Design review of the part shown in the three views and the two pictorial views. Dimensions are in mm from the part's minimum x, y and z. A direction names the side the tool comes from. Give positions to 0.01 mm unless a question says otherwise; leave off trailing zeros. Order: outer loops, then holes, each group sorted by start corner. A loop starts at its lowest first (then second) coordinate and runs counter-clockwise, first axis right, second up.
Item 1: Machinability: for the marked faces 1 and 2, which of the approach directions +Z, -Z, +X, -X, +Y, -Y give a long, thin tool a straight path to every point of the face, cutting with its end or side? Answer none if there is none.
Item 2: For P1, Ø8, axis at y = 17.5, z = 5.5, coming from the -X side; P2, Ø2, axis at x = 24.5, y = 38.5, coming from the +Z side; P3, Ø2, axis at x = 40, y = 11.5, coming from the +Z side, all flat-tipped, find the tip position at first contact; note any pin that passes through.
Item 3: Consider section A-A (x = 44). Give the boundary of the cut face in (y, z), plus the area to 3 significant figures.
Item 4: Consider section C-C (z = 19.25). Give the boundary of the cut face in (x, y) (1 decimal).
Item 5: For probe 1 along Z at (x, y) = (38, 24.5); probe 2 along Z at (x, y) = (8.5, 33.5) (1 decimal); probe 3 along X at (y, z) = (21.5, 24) (1 decimal), list the stretches that pass through material, from the lowest coordinate up.
Item 6: The part is to be moulded in two halves that separate along X. For the marked faces 3, 4 and 5, say which applies: released by +X, released by -X, zero draft, split by the parting line, or undercut.
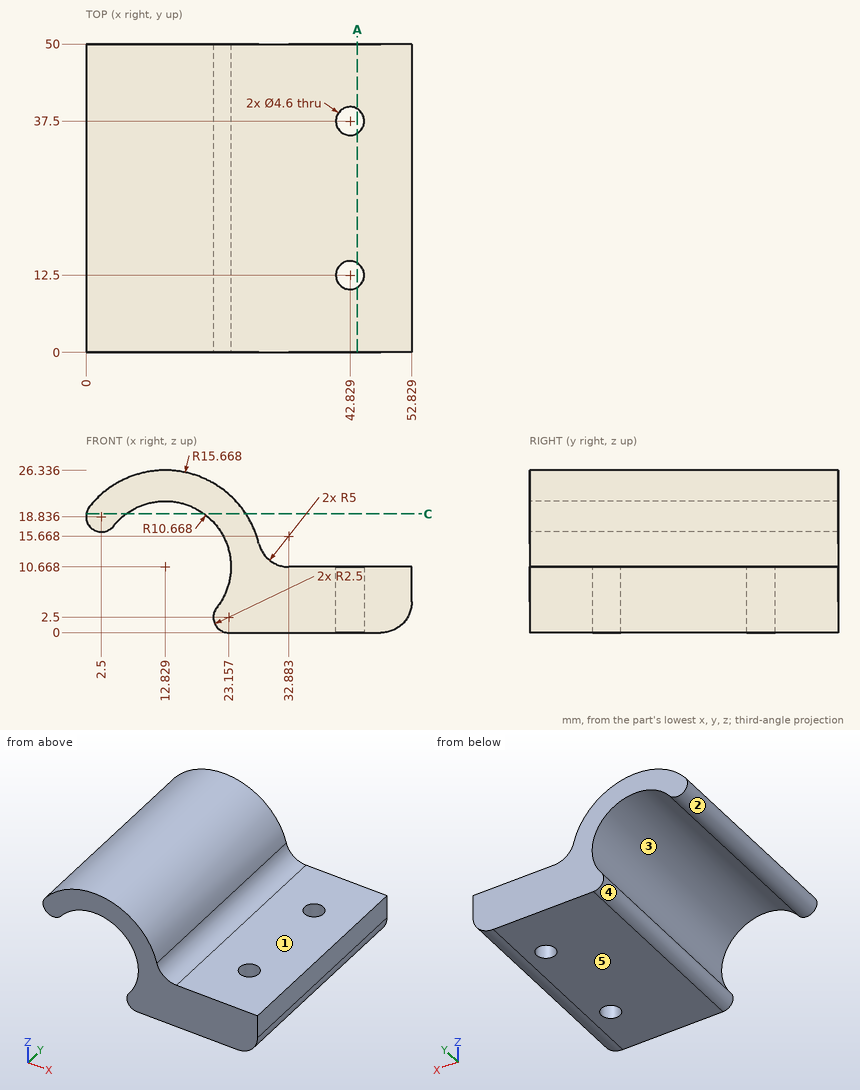
Resolved:
1. face 1: +Z, +X, +Y, -Y
1. face 2: +Y, -Y
2. P1: stops at x = 20.66
2. P2: stops at z = 22.14
2. P3: stops at z = 10.67
3. outline: (0, 0) - (10.52, 0) - (10.52, 10.67) - (0, 10.67) - close; (14.48, 0) - (35.52, 0) - (35.52, 10.67) - (14.48, 10.67) - close; (39.48, 0) - (50, 0) - (50, 10.67) - (39.48, 10.67) - close
3. area: 449 mm2
4. outline: (0, 0) - (6.5, 0) - (6.5, 50) - (0, 50) - close; (19.2, 0) - (25.9, 0) - (25.9, 50) - (19.2, 50) - close
5. probe 1: z = 0 to 10.67
5. probe 2: z = 20.4 to 25.7
5. probe 3: x = 4.6 to 21.1
6. face 3: undercut
6. face 4: released by -X
6. face 5: zero draft
